Read the model definition and answer for the solid it produces. Units are mm, in the model's axes. Coordinates: 2 decimals unless noted, no trailing zeros. Write each loop counter-clockwise with the first axis right and the second up, starting at its lowest first coordinate (ties: lowest second). Pieces come first, ordered by that corner, then holes.
1) The part is cut by section A-A (y = 85). Determine the outline of the cut face in (x, z).
2) Find the intervals of material crossed by line 1 (Z direction, x = 2.95, y = 13.5), in increasing order.
3) Each of these flat-tipped pins is pushed along its axis until it touches: pin 1 Ø1.5 at (x, z) = (2, -198) entering from -Y; pin 2 Ø1.5 at (x, z) = (1, -179) entering from -Y; pin 3 Ø1.5 at (x, z) = (1, -2) entering from +Y; pin 4 Ø1 at (x, y) = (2.5, 121.5) entering from -Z. Where does it stop, or does it pass through?
Autodesk Inventor part; units mm, degrees
ref_plane "YZ Plane" through (0, 0, 0) normal (1, 0, 0) x (0, 1, 0)
ref_plane "XZ Plane" through (0, 0, 0) normal (0, 1, 0) x (-1, 0, 0)
ref_plane "XY Plane" through (0, 0, 0) normal (0, 0, 1) x (1, 0, 0)
sketch "Sketch2" plane through (0, 0, 0) normal (1, 0, 0) x (0, 1, 0)
  line L0 (250, 0) -> (250, -200)
  line L1 (250, -200) -> (0, -200)
  line L2 (0, -200) -> (0, 0)
  line L3 (0, 0) -> (0, -3)
  line L4 (0, -3) -> (30, -3)
  line L5 (30, -3) -> (30, 0)
  line L6 (30, 0) -> (60, 0)
  line L7 (60, 0) -> (60, -3)
  line L8 (60, -3) -> (90, -3)
  line L9 (90, -3) -> (90, 0)
  line L10 (90, 0) -> (120, 0)
  line L11 (120, 0) -> (120, -3)
  line L12 (120, -3) -> (150, -3)
  line L13 (150, -3) -> (150, 0)
  line L14 (150, 0) -> (180, 0)
  line L15 (180, 0) -> (180, -3)
  line L16 (180, -3) -> (210, -3)
  line L17 (210, -3) -> (210, 0)
  line L18 (210, 0) -> (240, 0)
  line L19 (240, 0) -> (240, -3)
  line L20 (240, -3) -> (250, -3)
  line L21 (0, -100) -> (250, -100)
  line L22 (0, -197) -> (30, -197)
  line L23 (30, -197) -> (30, -200)
  line L24 (30, -200) -> (60, -200)
  line L25 (60, -200) -> (60, -197)
  line L26 (60, -197) -> (90, -197)
  line L27 (90, -197) -> (90, -200)
  line L28 (90, -200) -> (120, -200)
  line L29 (120, -200) -> (120, -197)
  line L30 (120, -197) -> (150, -197)
  line L31 (150, -197) -> (150, -200)
  line L32 (150, -200) -> (180, -200)
  line L33 (180, -200) -> (180, -197)
  line L34 (180, -197) -> (210, -197)
  line L35 (210, -197) -> (210, -200)
  line L36 (210, -200) -> (240, -200)
  line L37 (240, -200) -> (240, -197)
  line L38 (240, -197) -> (250, -197)
  dimension "d44" = 200
  dimension "d45" = 250
  dimension "d46" = 3
  dimension "d47" = 30
  dimension "d48" = 3
  dimension "d49" = 30
  dimension "d50" = 3
  dimension "d51" = 30
  dimension "d52" = 3
  dimension "d53" = 30
  dimension "d54" = 3
  dimension "d55" = 30
  dimension "d56" = 3
  dimension "d57" = 30
  dimension "d58" = 3
  dimension "d59" = 30
  dimension "d60" = 3
  dimension "d61" = 30
  dimension "d62" = 3
  dimension "d63" = 10
  dimension "d64" = 90
extrude "Extrusion2" add sketch "Sketch2" along normal blind 3 contours L0 L21 L2 L4 L5 L6 L7 L8 L9 L10 L11 L12 L13 L14 L15 L16 L17 L18 L19 L20 | L0 L38 L37 L1 L35 L34 L33 L31 L30 L29 L27 L26 L25 L23 L22 L2 L21
properties part number "Q side 2" material "ABS Plastic"
Reported:
1. outline: (0, -197) - (3, -197) - (3, -3) - (0, -3) - close
2. line 1: z = -197 to -3
3. pin 1: stops at y = 30
3. pin 2: stops at y = 0
3. pin 3: stops at y = 240
3. pin 4: stops at z = -197
